Read the model definition and answer for the solid it produces. Units are mm, in the model's axes. A direction names the side the tool comes from. Give positions to 0.01 mm unless a question says otherwise; leave off trailing zeros. Loops run counter-clockwise (first coordinate to the right, second up) from the corner with the lowest first, then second, coordinate; pieces in that order, holes last. Notation, with made-up numbers: (71, 42) - (111, 42) arc R17 cw to (111, 67) - close; hole circle Ø9 at (8.5, 1.5). An arc over 180 degrees is marked (long way). Use a Markdown table: item, result. Add a question column.
Item 1: Consider probe 1 along Z at (x, y) = (-26, 0); probe 2 along Y at (x, z) = (0, -17.25); probe 3 along Z at (x, y) = (7.5, -14.5). Determine where each line is inside the solid, lowest interval first. Write a range as [from, to].
Item 2: Which of the six approach directions +Z, -Z, +X, -X, +Y, -Y give full straight-line access (tool end or side, diameter ignored) to faces 1 (the face through (0, -8.03, -5)), 2 (the face through (0, 13, -10.2)), 3 (the face through (-20.14, -0.33, -2.52))?
Item 3: A cutting plane is placed at D-D (z = -27). Determine the outline of the cut face in (x, y).
Item 4: A cutting plane is placed at C-C (z = -5). Determine the outline of the cut face in (x, y), plus the area to 3 significant figures.
Item 5: Each of these flat-tipped pins is pushed along its axis until it touches: P1, Ø12, axis at y = -19.5, z = -24.5, coming from the -X side; P2, Ø5, axis at x = 0, z = -3, coming from the -Y side; P3, Ø1, axis at y = 19, z = -24, coming from the +X side. Where does it stop, or does it pass through?
Item 6: For a pull along X with two mould halves and no side action, classify faces 4 (the face through (25.9, 19.8, -17.8)), 5 (the face through (-10, 29, -35.2)), 6 (the face through (9, 26, -32.2)) as +X half, -X half, draft (parallel to the pull), parting line (faces both ways), or undercut.
Item 7: A cutting plane is placed at A-A (y = 0). Determine the outline of the cut face in (x, z), plus the area to 3 significant figures.
Item 8: A cutting plane is placed at B-B (x = 0). Determine the outline of the cut face in (y, z).
from build123d import *

# Parameters (mm, degrees)
F3_DEPTH        = 25
F4_R            = 2.5
F5_DEPTH        = 24.571
F5_COPIES_COUNT = 2
F5_COPIES_ANGLE = 270


# Not quite as in the source:
# - a pattern or mirror of a feature is missing from the dataset's text; its kind, count and spacing are read off the source's solid


with BuildPart() as f1:
    # F0 (on Front) → F1 (revolve)
    with BuildSketch(Plane.XZ):
        Polygon((0, -10.2), (0, 0), (-32.6, 0), (-32.6, -35.2), (-30.25, -35.2), (-27.25, -32.2), (-29.6, -32.2), (-29.6, -10.2), align=None)
    revolve(axis=Axis((0, 0, -5.1), (0, 0, 1)))

    # F2 (on face) → F3 (cut)
    with BuildSketch(Plane.XY):
        with BuildLine():
            ThreePointArc((8.03, 6.03), (7.4442135624, 7.4442135624), (6.03, 8.03))
            Line((6.03, 8.03), (-6.03, 8.03))
            ThreePointArc((-6.03, 8.03), (-7.4442135624, 7.4442135624), (-8.03, 6.03))
            Line((-8.03, 6.03), (-8.03, -6.03))
            ThreePointArc((-8.03, -6.03), (-7.4442135624, -7.4442135624), (-6.03, -8.03))
            Line((-6.03, -8.03), (6.03, -8.03))
            ThreePointArc((6.03, -8.03), (7.4442135624, -7.4442135624), (8.03, -6.03))
            Line((8.03, -6.03), (8.03, 6.03))
        make_face()
    extrude(amount=-F3_DEPTH, mode=Mode.SUBTRACT)

    # F4 (on face) → F5 (cut, through all)
    with BuildSketch(Plane.YZ.offset(-8.03)):
        with Locations((0, -5)):
            Circle(F4_R)
    f5 = extrude(amount=-F5_DEPTH, mode=Mode.SUBTRACT)

    # F5_copies: F5 ×2 about axis
    f5_copies_axis = Axis((0, 0, 0), (0, 0, 1))
    for i in range(1, F5_COPIES_COUNT):
        add(f5.rotate(f5_copies_axis, i * F5_COPIES_ANGLE / (F5_COPIES_COUNT - 1)), mode=Mode.SUBTRACT)


solid = f1.part
Geometry says:
| question | item | result |
|---|---|---|
| 1 | probe 1 | [-10.2, -7.5], [-2.5, 0] |
| 1 | probe 2 | [-32.6, -29.6], [29.6, 32.6] |
| 1 | probe 3 | [-10.2, 0] |
| 2 | face 1 | +Z, -Z |
| 2 | face 2 | none |
| 2 | face 3 | -X |
| 3 | outline | circle Ø65.2 at (0, 0); hole circle Ø59.2 at (0, 0) |
| 4 | outline | (-32.5, -2.5) arc R32.6 ccw (long way) to (2.5, 32.5) - (2.5, 8.03) - (6.03, 8.03) arc R2 cw to (8.03, 6.03) - (8.03, -6.03) arc R2 cw to (6.03, -8.03) - (-6.03, -8.03) arc R2 cw to (-8.03, -6.03) - (-8.03, -2.5) - close; (-32.5, 2.5) - (-8.03, 2.5) - (-8.03, 6.03) arc R2 cw to (-6.03, 8.03) - (-2.5, 8.03) - (-2.5, 32.5) arc R32.6 ccw to start |
| 4 | area | 2,840 mm² |
| 5 | P1 | x = -29.67 |
| 5 | P2 | y = -32.6 |
| 5 | P3 | x = 26.84 |
| 6 | face 4 | parting line |
| 6 | face 5 | draft |
| 6 | face 6 | undercut |
| 7 | outline | (-32.6, -35.2) - (-30.25, -35.2) - (-27.25, -32.2) - (-29.6, -32.2) - (-29.6, -10.2) - (-8.03, -10.2) - (-8.03, -7.5) - (-32.6, -7.5) - close; (-32.6, -2.5) - (-8.03, -2.5) - (-8.03, 0) - (-32.6, 0) - close; (8.03, -10.2) - (29.6, -10.2) - (29.6, -32.2) - (27.25, -32.2) - (30.25, -35.2) - (32.6, -35.2) - (32.6, 0) - (8.03, 0) - close |
| 7 | area | 533 mm² |
| 8 | outline | (-32.6, -35.2) - (-30.25, -35.2) - (-27.25, -32.2) - (-29.6, -32.2) - (-29.6, -10.2) - (-8.03, -10.2) - (-8.03, 0) - (-32.6, 0) - close; (8.03, -10.2) - (29.6, -10.2) - (29.6, -32.2) - (27.25, -32.2) - (30.25, -35.2) - (32.6, -35.2) - (32.6, -7.5) - (8.03, -7.5) - close; (8.03, -2.5) - (32.6, -2.5) - (32.6, 0) - (8.03, 0) - close |
